from build123d import *

# Parameters (mm, degrees)
SKETCH_1_W      = 10
SKETCH_1_H      = 3
SKETCH_1_W_2    = 0.64
SKETCH_1_H_2    = 0.64
EXTRUDE_1_DEPTH = 6
SKETCH_2_W      = 10
SKETCH_2_H      = 3
SKETCH_2_R      = 0.5
EXTRUDE_2_DEPTH = 2
CHAMFER_1_SIZE  = 0.5


with BuildPart() as part:
    # Эскиз1 → Бобышка-Вытянуть1 (new body)
    with BuildSketch(Plane(origin=(0, 0, 0), x_dir=(1, 0, 0), z_dir=(0, 1, 0))):
        Rectangle(SKETCH_1_W, SKETCH_1_H)
        with Locations((-3.81, 0)):
            Rectangle(SKETCH_1_W_2, SKETCH_1_H_2, mode=Mode.SUBTRACT)
        with Locations((3.81, 0)):
            Rectangle(SKETCH_1_W_2, SKETCH_1_H_2, mode=Mode.SUBTRACT)
        with Locations((-1.27, 0)):
            Rectangle(SKETCH_1_W_2, SKETCH_1_H_2, mode=Mode.SUBTRACT)
        with Locations((1.27, 0)):
            Rectangle(SKETCH_1_W_2, SKETCH_1_H_2, mode=Mode.SUBTRACT)
    extrude(amount=EXTRUDE_1_DEPTH)

    # Эскиз2 → Бобышка-Вытянуть2 (add)
    with BuildSketch(Plane(origin=(0, 6, 0), x_dir=(1, 0, 0), z_dir=(0, 1, 0))):
        Rectangle(SKETCH_2_W, SKETCH_2_H)
        with Locations((-3.81, 0)):
            Circle(SKETCH_2_R, mode=Mode.SUBTRACT)
        with Locations((-1.27, 0)):
            Circle(SKETCH_2_R, mode=Mode.SUBTRACT)
        with Locations((1.27, 0)):
            Circle(SKETCH_2_R, mode=Mode.SUBTRACT)
        with Locations((3.81, 0)):
            Circle(SKETCH_2_R, mode=Mode.SUBTRACT)
    extrude(amount=EXTRUDE_2_DEPTH)

    # Фаска1
    chamfer_1_edges = [part.edges().sort_by_distance(p)[0] for p in [
        (5, 4, 1.5),
        (-5, 4, 1.5),
        (-5, 4, -1.5),
        (5, 4, -1.5),
    ]]
    chamfer(chamfer_1_edges, length=CHAMFER_1_SIZE)


solid = part.part
Could you check a few things on this model? Use its own coordinates, in mm. A direction names the side the tool comes from. Give positions to 0.01 mm unless a question says otherwise; leave off trailing zeros. Order: outer loops, then holes, each group sorted by start corner. A loop starts at its lowest first (then second) coordinate and runs counter-clockwise, first axis right, second up.
Item 1: If we section it at A-A, the plane x = 1.27: Write out the boundary of the cut face in (y, z), plus the area to 3 significant figures.
Item 2: I'm going to push a flat-ended pin straight in: pin 1 (0.8 mm diameter, centred on x = -1.5, z = 0, fed in from +Y). Where does the tip first touch, or does it pass through?
Item 3: For faces 1 (the face through (0, 0, 0)), 2 (the face through (3.31, 6.99, -0.02)), which set-ups out of +Z, -Z, +X, -X, +Y, -Y let a thin tool reach every point of the face, with its end or its side?
Item 4: If we section it at B-B, the plane y = 6.5: Write out the boundary of the cut face in (x, z), plus the area to 3 significant figures.
Item 5: If we mould it in two halves opening along Z, with no side actions, what happens to faces 3 (the face through (0, 4, 1.5)), 4 (the face through (0, 4, -1.5)), 5 (the face through (-0.808, 6.986, 0.192)), 6 (the face through (-5, 4, 0))? For each: pulls with the +Z half, pulls with the -Z half, needs draft (parallel to the pull), parting line crosses it, or undercut.
Item 6: If we section it at D-D, the plane x = 4: Write out the boundary of the cut face in (y, z), plus the area to 3 significant figures.
Item 7: I need wall thicknesses on line 1 (X direction, y = 7.2, z = 0); line 2 (X direction, y = 1.5, z = -0.2); line 3 (Z direction, x = 3.81, y = 6.95). Which ranges of each line are inside material? Lowest first, please.
Item 8: If we section it at C-C, the plane z = 0: Count the separate pieces of the cut face and the enclosed holes in it, plus the area to 3 significant figures.
Values:
1. outline: (0, -1.5) - (8, -1.5) - (8, -0.5) - (6, -0.5) - (6, -0.32) - (0, -0.32) - close; (0, 0.32) - (6, 0.32) - (6, 0.5) - (8, 0.5) - (8, 1.5) - (0, 1.5) - close
1. area: 18.2 mm2
2. pin 1: stops at y = 8
3. face 1: +Z, -Z, +X, -X, -Y
3. face 2: +Y
4. outline: (-5, -1) - (-4.5, -1.5) - (4.5, -1.5) - (5, -1) - (5, 1) - (4.5, 1.5) - (-4.5, 1.5) - (-5, 1) - close; hole circle Ø1 at (-3.81, 0); hole circle Ø1 at (-1.27, 0); hole circle Ø1 at (1.27, 0); hole circle Ø1 at (3.81, 0)
4. area: 26.4 mm2
5. face 3: pulls with the +Z half
5. face 4: pulls with the -Z half
5. face 5: undercut
5. face 6: needs draft
6. outline: (0, -1.5) - (8, -1.5) - (8, -0.46) - (6, -0.46) - (6, -0.32) - (0, -0.32) - close; (0, 0.32) - (6, 0.32) - (6, 0.46) - (8, 0.46) - (8, 1.5) - (0, 1.5) - close
6. area: 18.3 mm2
7. line 1: x = -5 to -4.31, -3.31 to -1.77, -0.77 to 0.77, 1.77 to 3.31, 4.31 to 5
7. line 2: x = -5 to -4.13, -3.49 to -1.59, -0.95 to 0.95, 1.59 to 3.49, 4.13 to 5
7. line 3: z = -1.5 to -0.5, 0.5 to 1.5
8. separate pieces: 5
8. enclosed holes: 0
8. area: 56.6 mm2
